Could you check a few things on this model? Use its own coordinates, in mm. Coordinates: 2 decimals unless noted, no trailing zeros. Loops run counter-clockwise (first coordinate to the right, second up) from the corner with the lowest first, then second, coordinate; pieces in that order, holes last. Notation, with made-up numbers: (21, 5.5) - (60, 5.5) arc R17 ccw to (60, 10.5) - close; hole circle Ø1 at (75.25, -29). An arc over 180 degrees is marked (long way). One line per item, written item: value. Start each with the question number.
(1) If I drill on line 1 along Z through (x, y) = (153.5, 877); line 2 along Z through (x, y) = (219, -646.5); line 3 along Y through (x, z) = (107, 100.5), over which ranges is the centre line in solid material (lowest first)? Write a range as from..to.
(2) If we section it at A-A on x = 54.5: Write out the boundary of the cut face in (y, z).
(3) If we section it at B-B on x = 201.5: Write out the boundary of the cut face in (y, z), then the cut area to 3 significant figures.
(4) I'm going to push flat-ended pins straight in: P1, Ø12, axis at x = 27.5, z = 698.5, coming from the +Y side; P2, Ø2, axis at x = 139.5, y = -509, coming from the -Z side; P3, Ø10, axis at x = 50.5, z = 296, coming from the -Y side. Where does each tip first touch, or does it pass through?
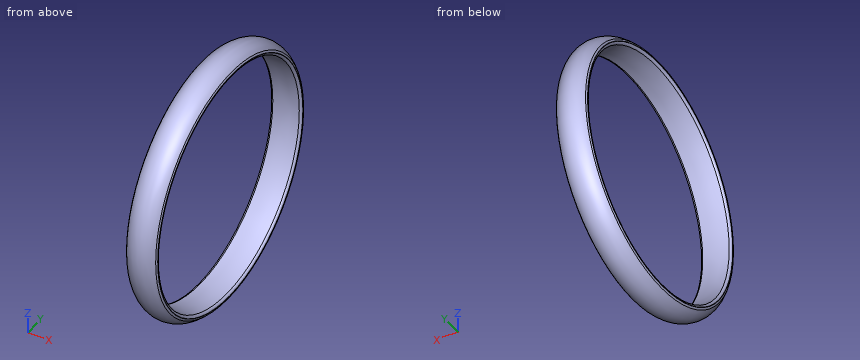
```python
from build123d import *


with BuildPart() as part:
    # Sketch → Revolution (revolve)
    with BuildSketch(Plane.XY):
        with BuildLine():
            Line((0, -982.510836), (0, -985.611786))
            ThreePointArc((0, -985.611786), (1.676589, -994.612814), (6.481481, -1002.406561))
            ThreePointArc((6.481481, -1002.406561), (125, -1054.92), (243.518519, -1002.406561))
            ThreePointArc((243.518519, -1002.406561), (248.323411, -994.612814), (250, -985.611786))
            Line((250, -982.510836), (250, -985.611786))
            ThreePointArc((250, -982.510836), (245.12505, -969.425238), (232.876712, -962.718804))
            ThreePointArc((232.876712, -962.718804), (125, -954.92), (17.123288, -962.718804))
            ThreePointArc((17.123288, -962.718804), (4.87495, -969.425238), (0, -982.510836))
        make_face()
    revolve(axis=Axis((0, 0, 0), (1, 0, 0)))


solid = part.part
```
Values:
1. line 1: z = -581.67..-379.18, 379.18..581.67
1. line 2: z = -794.62..-710.8, 710.8..794.62
1. line 3: y = -1049.1..-949.83, 949.83..1049.1
2. outline: circle Ø2077.1 at (0, 0); hole circle Ø1916.48 at (0, 0)
3. outline: circle Ø2070.89 at (0, 0); hole circle Ø1917.66 at (0, 0)
3. area: 480,000 mm2
4. P1: stops at y = 753.99
4. P2: stops at z = -923.81
4. P3: stops at y = -996.38
